CAD build for the part. Positions are in the model's coordinates, mm. A direction names the side the tool comes from. Coordinates: 2 decimals unless noted, no trailing zeros. Write each loop counter-clockwise with the first axis right and the second up, starting at its lowest first coordinate (ties: lowest second). Pieces come first, ordered by that corner, then holes. Notation, with made-up numbers: (63.5, 30) - (76.5, 30) arc R12 cw to (76.5, 41) - close; hole circle Ø8 at (-30, 42). An arc over 180 degrees is marked (long way). One line per question, with ' | ' between items. Start each with the question number.
1. Band-saw the part on D-D, the plane z = -15. Write the cut outline in (x, y), then the cut area to 3 significant figures.
2. Band-saw the part on C-C, the plane y = 11.75. Write the cut outline in (x, z).
3. Two-plate mould, pull along X, no slides. Class faces 1 (the flat face through (22.5, 13, -23)), 2 (the flat face through (0, 9, -23)), 3 (the flat face through (13, 9, -45)): +X half, -X half, draft (parallel to the pull), parting line (faces both ways), or undercut.
4. Band-saw the part on B-B, the plane x = 12.5. Write the cut outline in (y, z), then the cut area to 3 significant figures.
5. Flat gauge pins, fed straight in: P1, Ø0.6, axis at x = 13, z = -43.5, coming from the +Y side; P2, Ø3, axis at x = 14.5, z = -21.5, coming from the +Y side; P3, Ø8, axis at x = 12.5, z = -32.75, coming from the +Y side. Where does each tip first touch, or does it go through?
6. Band-saw the part on A-A, the plane z = -32.75. Write the cut outline in (x, y).
7. Probe line 1 (X direction, y = 4, z = -32.75); line 2 (X direction, y = 0.4, z = -32.75); line 3 (Z direction, x = 11.5, y = 12.75). List the from-to ranges inside material, lowest first.
8. Which spindle directions (+Z, -Z, +X, -X, +Y, -Y) get a long thin tool onto all of the face, cutting with end or side? Do faces 4 (the flat face through (12, 12, -43)), 5 (the flat face through (12, 13, -44)), 6 (the cylindrical face through (11.59, 0.51, -33.94)). Say none if no direction does.
from build123d import *

# Parameters (mm, degrees)
SKETCH1_W          = 25
SKETCH1_H          = 45
BASE_DEPTH         = 13
SKETCH2_W          = 20
SKETCH2_H          = 41
SEAT_DEPTH         = 5
SKETCH3_R          = 1.5
SCREWHOLE_DEPTH    = 8
SKETCH4_R          = 6.5
SCREWINSET_DEPTH   = 7
SEATSECURITY_DEPTH = 5


with BuildPart() as part:
    # Sketch1 → Base (new body)
    with BuildSketch(Plane(origin=(0, 0, 0), x_dir=(1, 0, 0), z_dir=(0, 1, 0))):
        with Locations((12.5, 22.5)):
            Rectangle(SKETCH1_W, SKETCH1_H)
    extrude(amount=BASE_DEPTH)

    # Sketch2 → Seat (cut)
    with BuildSketch(Plane(origin=(0, 13, 0), x_dir=(1, 0, 0), z_dir=(0, 1, 0))):
        with Locations((12.5, 22.5)):
            Rectangle(SKETCH2_W, SKETCH2_H)
    extrude(amount=-SEAT_DEPTH, mode=Mode.SUBTRACT)

    # Sketch3 → ScrewHole (cut)
    with BuildSketch(Plane(origin=(0, 8, 0), x_dir=(1, 0, 0), z_dir=(0, 1, 0))):
        with Locations(Location((12.5, 32.75, 0), (0, 0, 270))):
            Circle(SKETCH3_R)
    extrude(amount=-SCREWHOLE_DEPTH, mode=Mode.SUBTRACT)

    # Sketch4 → ScrewInset (cut)
    with BuildSketch(Plane(origin=(0, 8, 0), x_dir=(1, 0, 0), z_dir=(0, 1, 0))):
        with Locations(Location((12.5, 32.75, 0), (0, 0, 270))):
            Circle(SKETCH4_R)
    extrude(amount=-SCREWINSET_DEPTH, mode=Mode.SUBTRACT)

    # Sketch6 → SeatSecurity (add)
    with BuildSketch(Plane(origin=(0, 13, 0), x_dir=(1, 0, 0), z_dir=(0, 1, 0))):
        Polygon((2.5, 2), (2.5, 43), (8.5, 43), (8.5, 45), (0, 45), (0, 0), (25, 0), (25, 45), (16.5, 45), (16.5, 43), (22.5, 43), (22.5, 2), align=None)
    extrude(amount=SEATSECURITY_DEPTH)


solid = part.part
Filled in:
1) outline: (0, 0) - (25, 0) - (25, 18) - (22.5, 18) - (22.5, 8) - (2.5, 8) - (2.5, 18) - (0, 18) - close | area: 250 mm²
2) outline: (0, -45) - (25, -45) - (25, 0) - (0, 0) - close; hole (2.5, -43) - (22.5, -43) - (22.5, -2) - (2.5, -2) - close
3) face 1: undercut | face 2: -X half | face 3: draft
4) outline: (0, -45) - (13, -45) - (13, -43) - (8, -43) - (8, -39.25) - (1, -39.25) - (1, -34.25) - (0, -34.25) - close; (0, -31.25) - (1, -31.25) - (1, -26.25) - (8, -26.25) - (8, -2) - (18, -2) - (18, 0) - (0, 0) - close | area: 296 mm²
5) P1: stops at y = 13 | P2: stops at y = 8 | P3: stops at y = 1
6) outline: (0, 0) - (11, 0) - (11, 1) - (6, 1) - (6, 8) - (2.5, 8) - (2.5, 18) - (0, 18) - close; (14, 0) - (25, 0) - (25, 18) - (22.5, 18) - (22.5, 8) - (19, 8) - (19, 1) - (14, 1) - close
7) line 1: x = 0 to 6, 19 to 25 | line 2: x = 0 to 11, 14 to 25 | line 3: z = -45 to -43, -2 to 0
8) face 4: +Y | face 5: -Z, +Y | face 6: +Y, -Y
